Can you work these out from the model? Positions are in its coordinate system, mm. Face numbers are marked on the shaded views. A direction names the side the tool comes from. Coordinates: 2 decimals unless noted, no trailing zeros. Order: outer loops, then holes, each group sorted by start corner. A loop starts at its lowest first (then second) coordinate and runs counter-clockwise, first axis right, second up. Notation, with made-up numbers: (76, 56) -> (115, 56) arc R36 ccw to (115, 93) -> close; hole circle Ø11 at (73, -18.75). An arc over 180 degrees is marked (long way). Answer in a Markdown table with one row per item. Add a question column.
1. Will these pins go through, and if not, where does the flat tip stop? pin 1 (3 mm diameter, centred on x = -2.5, z = 5.5, fed in from -Y); pin 2 (3 mm diameter, centred on x = 2.5, y = -33.5, fed in from +Z); pin 3 (6 mm diameter, centred on x = -5, y = -47.5, fed in from -Z).
2. Imagine slicing it at A-A on x = 0. Write out the boundary of the cut face in (y, z).
3. Imagine slicing it at B-B on y = 0. Write out the boundary of the cut face in (x, z), plus the area to 4 significant figures.
4. Imagine slicing it at C-C on z = 4.75. Write out the boundary of the cut face in (x, y).
5. On a 3-axis mill with a long thin cutter (end or side, diameter ignored), from which of +Z, -Z, +X, -X, +Y, -Y can I reach the whole of each face in a straight line? I mean the marked faces 1 and 2. Say none if no direction works.
6. If I drill on line 1 along X through (y, z) = (0, 7); line 2 along Y through (x, z) = (-8.75, 4.25); line 3 along X through (y, z) = (-13, 4.25), over which ranges is the centre line in solid material (lowest first)? Write a range as [from, to].
7. Imagine slicing it at D-D on x = 8.75. Write out the boundary of the cut face in (y, z).
from build123d import *

# Parameters (mm, degrees)
CROQUIS1_R               = 10
SALIENTE_EXTRUIR1_DEPTH  = 3
CROQUIS2_R               = 11.5
CROQUIS2_R_2             = 10
SALIENTE_EXTRUIR3_DEPTH  = 8
SALIENTE_EXTRUIR4_START  = 3
CROQUIS3_R               = 11.5
CROQUIS3_R_2             = 10
SALIENTE_EXTRUIR4_DEPTH  = 3
SALIENTE_EXTRUIR5_DEPTH  = 8
CROQUIS11_W              = 0.560242515
CROQUIS11_H              = 6
CORTAR_EXTRUIR3_DEPTH    = 8
CROQUIS12_W              = 2.5
CROQUIS12_H              = 0.622045166
SALIENTE_EXTRUIR6_DEPTH  = 3
CROQUIS13_W              = 5
CROQUIS13_H              = 50.27502784
SALIENTE_EXTRUIR7_DEPTH  = 8
CROQUIS15_W              = 2
CROQUIS15_H              = 50.27502784
CORTAR_EXTRUIR4_DEPTH    = 8
SALIENTE_EXTRUIR8_DEPTH  = 7
CROQUIS21_R              = 10
SALIENTE_EXTRUIR9_DEPTH  = 7
CROQUIS22_R              = 5
CORTAR_EXTRUIR5_DEPTH    = 30
CROQUIS23_R              = 10
SALIENTE_EXTRUIR10_DEPTH = 1.25
CORTAR_EXTRUIR6_START    = -1.5
CROQUIS24_R              = 10
CORTAR_EXTRUIR6_DEPTH    = 1.5
SALIENTE_EXTRUIR11_START = -3
CROQUIS25_R              = 13
SALIENTE_EXTRUIR11_DEPTH = 3
CORTAR_EXTRUIR14_START   = -10
CROQUIS30_R              = 10
CORTAR_EXTRUIR14_DEPTH   = 10
CROQUIS31_R              = 11.5
CROQUIS31_R_2            = 10
SALIENTE_EXTRUIR12_DEPTH = 7.75


with BuildPart() as part:
    # Croquis1 → Saliente-Extruir1 (new body)
    with BuildSketch(Plane.XY):
        Circle(CROQUIS1_R)
    extrude(amount=SALIENTE_EXTRUIR1_DEPTH)



with BuildPart() as body_2:
    # Croquis2 → Saliente-Extruir3 (new body)
    with BuildSketch(Plane.XY.offset(3)):
        Circle(CROQUIS2_R)
        Circle(CROQUIS2_R_2, mode=Mode.SUBTRACT)
    extrude(amount=SALIENTE_EXTRUIR3_DEPTH)


with BuildPart() as part_1:
    add(part.part)

    add(body_2.part)  # Saliente-Extruir4 merges body 2
    # Croquis3 → Saliente-Extruir4 (add)
    with BuildSketch(Plane(origin=(0, 0, 3), x_dir=(-1, 0, 0), z_dir=(0, 0, -1)).offset(SALIENTE_EXTRUIR4_START)):
        with Locations(Location((0, 0, 0), (0, 0, 180))):
            Circle(CROQUIS3_R)
        with Locations(Location((0, 0, 0), (0, 0, 180))):
            Circle(CROQUIS3_R_2, mode=Mode.SUBTRACT)
    extrude(amount=-SALIENTE_EXTRUIR4_DEPTH)

    # Croquis12 → Saliente-Extruir6 (add)
    with BuildSketch(Plane.XY.offset(3)):
        with Locations((-1.25, -11.188977417)):
            Rectangle(CROQUIS12_W, CROQUIS12_H)
        with Locations((1.25, -11.188977417)):
            Rectangle(CROQUIS12_W, CROQUIS12_H)
        Polygon((2.5, -11.5), (2.5, -61.5), (-2.5, -61.5), (-2.5, -11.5), (0, -11.5), align=None)
    extrude(amount=-SALIENTE_EXTRUIR6_DEPTH)

    # Croquis13 → Saliente-Extruir7 (add)
    with BuildSketch(Plane.XY.offset(3)):
        with Locations((0, -36.36248608)):
            Rectangle(CROQUIS13_W, CROQUIS13_H)
    extrude(amount=SALIENTE_EXTRUIR7_DEPTH)

    # Croquis15 → Cortar-Extruir4 (cut)
    with BuildSketch(Plane(origin=(2.5, 0, 0), x_dir=(0, 0, -1), z_dir=(1, 0, 0))):
        with Locations((-10, -36.36248608)):
            Rectangle(CROQUIS15_W, CROQUIS15_H)
        with Locations((-1, -36.36248608)):
            Rectangle(CROQUIS15_W, CROQUIS15_H)
    extrude(amount=-CORTAR_EXTRUIR4_DEPTH, mode=Mode.SUBTRACT)

    # Croquis16 → Saliente-Extruir8 (add)
    with BuildSketch(Plane.XY.offset(9)):
        Polygon((-2.5, -61.5), (-3.5, -61.5), (-3.5, -10.232955502), (3.5, -10.232955502), (3.5, -61.5), (2.5, -61.5), align=None)
    extrude(amount=-SALIENTE_EXTRUIR8_DEPTH)

    # Croquis21 → Saliente-Extruir9 (add)
    with BuildSketch(Plane(origin=(0, 0, 2), x_dir=(-1, 0, 0), z_dir=(0, 0, -1))):
        with Locations((0, -52.72497216)):
            Circle(CROQUIS21_R)
    extrude(amount=-SALIENTE_EXTRUIR9_DEPTH)

    # Croquis22 → Cortar-Extruir5 (cut)
    with BuildSketch(Plane(origin=(0, 0, 2), x_dir=(-1, 0, 0), z_dir=(0, 0, -1))):
        with Locations((0, -52.72497216)):
            Circle(CROQUIS22_R)
    extrude(amount=-CORTAR_EXTRUIR5_DEPTH, mode=Mode.SUBTRACT)

    # Croquis23 → Saliente-Extruir10 (add)
    with BuildSketch(Plane.XY.offset(11)):
        with BuildLine():
            Line((-2.5, -11.22497216), (2.5, -11.22497216))
            ThreePointArc((2.5, -11.22497216), (0, 11.5), (-2.5, -11.22497216))
        make_face()
        Circle(CROQUIS23_R, mode=Mode.SUBTRACT)
    extrude(amount=SALIENTE_EXTRUIR10_DEPTH)

    # Croquis24 → Cortar-Extruir6 (cut)
    with BuildSketch(Plane.XY.offset(12.25).offset(CORTAR_EXTRUIR6_START)):
        with BuildLine():
            Line((-2.5, -11.22497216), (2.5, -11.22497216))
            ThreePointArc((2.5, -11.22497216), (0, 11.5), (-2.5, -11.22497216))
        make_face()
        Circle(CROQUIS24_R, mode=Mode.SUBTRACT)
    extrude(amount=CORTAR_EXTRUIR6_DEPTH, mode=Mode.SUBTRACT)

    # Croquis25 → Saliente-Extruir11 (add)
    with BuildSketch(Plane.XY.offset(10.75).offset(SALIENTE_EXTRUIR11_START)):
        Circle(CROQUIS25_R)
        with BuildLine():
            ThreePointArc((2.5, -11.22497216), (0, 11.5), (-2.5, -11.22497216))
            Line((-2.5, -11.22497216), (2.5, -11.22497216))
        make_face(mode=Mode.SUBTRACT)
    extrude(amount=SALIENTE_EXTRUIR11_DEPTH)

    # Croquis30 → Cortar-Extruir14 (cut)
    with BuildSketch(Plane.XY.offset(3).offset(CORTAR_EXTRUIR14_START)):
        Circle(CROQUIS30_R)
    extrude(amount=CORTAR_EXTRUIR14_DEPTH, mode=Mode.SUBTRACT)

    # Croquis31 → Saliente-Extruir12 (add)
    with BuildSketch(Plane(origin=(0, 0, 0), x_dir=(-1, 0, 0), z_dir=(0, 0, -1))):
        with Locations(Location((0, 0, 0), (0, 0, 180))):
            Circle(CROQUIS31_R)
        with Locations(Location((0, 0, 0), (0, 0, 180))):
            Circle(CROQUIS31_R_2, mode=Mode.SUBTRACT)
    extrude(amount=-SALIENTE_EXTRUIR12_DEPTH)


with BuildPart() as body_2_2:
    # Croquis9 → Saliente-Extruir5 (new body)
    with BuildSketch(Plane.XY.offset(11)):
        Polygon((11.5, 0), (11.5, 3), (12.060242515, 3), (12.060242515, -3), (11.5, -3), align=None)
    extrude(amount=-SALIENTE_EXTRUIR5_DEPTH)

    # Croquis11 → Cortar-Extruir3 (cut)
    with BuildSketch(Plane.XY.offset(11)):
        with Locations((11.780121257, 0)):
            Rectangle(CROQUIS11_W, CROQUIS11_H)
    extrude(amount=-CORTAR_EXTRUIR3_DEPTH, mode=Mode.SUBTRACT)


solid = part_1.part
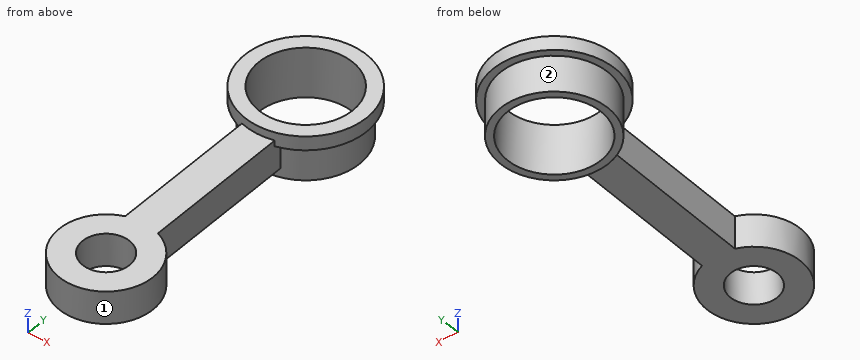
Answers follow:
| question | item | result |
|---|---|---|
| 1 | pin 1 | stops at y = -62.67 |
| 1 | pin 2 | stops at z = 9 |
| 1 | pin 3 | stops at z = 2 |
| 2 | outline | (-62.72, 2) -> (-57.72, 2) -> (-57.72, 9) -> (-62.72, 9) -> close; (-47.72, 2) -> (-11.5, 2) -> (-11.5, 0) -> (-10, 0) -> (-10, 10.75) -> (-13, 10.75) -> (-13, 9) -> (-47.72, 9) -> close; (10, 0) -> (11.5, 0) -> (11.5, 7.75) -> (13, 7.75) -> (13, 10.75) -> (10, 10.75) -> close |
| 3 | outline | (-13, 7.75) -> (-11.5, 7.75) -> (-11.5, 0) -> (-10, 0) -> (-10, 10.75) -> (-13, 10.75) -> close; (10, 0) -> (11.5, 0) -> (11.5, 7.75) -> (13, 7.75) -> (13, 10.75) -> (10, 10.75) -> close |
| 3 | area | 41.25 mm² |
| 4 | outline | (-3.5, -43.36) arc R10 ccw (long way) to (3.5, -43.36) -> (3.5, -10.95) arc R11.5 ccw (long way) to (-3.5, -10.95) -> close; hole circle Ø20 at (0, 0); hole circle Ø10 at (0, -52.72) |
| 5 | face 1 | +Z, -Z |
| 5 | face 2 | -Z |
| 6 | line 1 | x = [-11.5, -10], [10, 11.5] |
| 6 | line 2 | y = [-57.57, -47.88], [-7.46, -4.84], [4.84, 7.46] |
| 6 | line 3 | x = [-3.5, 3.5] |
| 7 | outline | (-57.57, 2) -> (-47.88, 2) -> (-47.88, 9) -> (-57.57, 9) -> close; (-9.61, 7.75) -> (-7.46, 7.75) -> (-7.46, 0) -> (-4.84, 0) -> (-4.84, 10.75) -> (-9.61, 10.75) -> close; (4.84, 0) -> (7.46, 0) -> (7.46, 7.75) -> (9.61, 7.75) -> (9.61, 10.75) -> (4.84, 10.75) -> close |
